```python
from build123d import *

# Parameters (mm, degrees)
SKETCH1_W               = 56
SKETCH1_H               = 4
BOSS_EXTRUDE1_DEPTH     = 168
SKETCH3_W               = 4
SKETCH3_H               = 32
BOSS_EXTRUDE4_DEPTH     = 4
LPATTERN2_COUNT         = 3
LPATTERN2_PITCH         = 50
MIRROR2_COPY_1_SKETCH_W = 4
MIRROR2_COPY_1_SKETCH_H = 32
MIRROR2_COPY_1_DEPTH    = 4
MIRROR2_COPY_2_SKETCH_W = 4
MIRROR2_COPY_2_SKETCH_H = 32
MIRROR2_COPY_2_DEPTH    = 4
SKETCH4_W               = 12
SKETCH4_H               = 4
BOSS_EXTRUDE5_DEPTH     = 4


with BuildPart() as part:
    # Sketch1 → Boss-Extrude1 (new body)
    with BuildSketch(Plane(origin=(0, 0, 0), x_dir=(1, 0, 0), z_dir=(0, 1, 0))):
        Rectangle(SKETCH1_W, SKETCH1_H)
    extrude(amount=BOSS_EXTRUDE1_DEPTH)

    # Sketch3 → Boss-Extrude4 (add, through all)
    with BuildSketch(Plane.XY.offset(2)):
        with Locations((-30, 34)):
            Rectangle(SKETCH3_W, SKETCH3_H)
    boss_extrude4 = extrude(amount=-BOSS_EXTRUDE4_DEPTH)

    # LPattern2: Boss-Extrude4 ×3
    with Locations(*[(0, i * LPATTERN2_PITCH, 0) for i in range(1, LPATTERN2_COUNT)]):
        add(boss_extrude4)

    # Mirror2: Boss-Extrude4 across plane
    add(boss_extrude4.mirror(Plane(origin=(0, 0, 0), x_dir=(0, 0, 1), z_dir=(1, 0, 0))))

    # Mirror2 copy 1 sketch → Mirror2 copy 1 (add, through all)
    with BuildSketch(Plane(origin=(0, 50, 2), x_dir=(-1, 0, 0), z_dir=(0, 0, 1))):
        with Locations((-30, -34)):
            Rectangle(MIRROR2_COPY_1_SKETCH_W, MIRROR2_COPY_1_SKETCH_H)
    extrude(amount=-MIRROR2_COPY_1_DEPTH)

    # Mirror2 copy 2 sketch → Mirror2 copy 2 (add, through all)
    with BuildSketch(Plane(origin=(0, 100, 2), x_dir=(-1, 0, 0), z_dir=(0, 0, 1))):
        with Locations((-30, -34)):
            Rectangle(MIRROR2_COPY_2_SKETCH_W, MIRROR2_COPY_2_SKETCH_H)
    extrude(amount=-MIRROR2_COPY_2_DEPTH)

    # Sketch4 → Boss-Extrude5 (add, through all)
    with BuildSketch(Plane.XY.offset(2)):
        with Locations((-22, 170)):
            Rectangle(SKETCH4_W, SKETCH4_H)
        with Locations((0, 170)):
            Rectangle(SKETCH4_W, SKETCH4_H)
        with Locations((22, 170)):
            Rectangle(SKETCH4_W, SKETCH4_H)
    boss_extrude5 = extrude(amount=-BOSS_EXTRUDE5_DEPTH)

    # Mirror3: Boss-Extrude5 across plane
    add(boss_extrude5.mirror(Plane.ZX.offset(84)))


solid = part.part
```
Can you work these out from the model? Positions are in its coordinate system, mm. A direction names the side the tool comes from. Give positions to 0.01 mm unless a question says otherwise; leave off trailing zeros. Loops run counter-clockwise (first coordinate to the right, second up) from the corner with the lowest first, then second, coordinate; pieces in that order, holes last. Notation, with made-up numbers: M -16,-9 L 15,-9 A26 cw 15,7 Z; hole C 37.5,89.25 d1. An arc over 180 degrees is marked long. Answer in a Markdown table with one row per item.
1. For pin 1 Ø2 at (y, z) = (-2, -0.5) entering from -X; pin 2 Ø2 at (x, z) = (31, 0.5) entering from +Y; pin 3 Ø1.2 at (x, z) = (30.5, 0) entering from -Y, each with a flat end and sliding along its axis, tell me the tip position at first contact or that it passes through.
Taken from the geometry:
| item | result |
|---|---|
| pin 1 | stops at x = -28 |
| pin 2 | stops at y = 150 |
| pin 3 | stops at y = 18 |
2. Suppose I cut it at A-A on x = -10. Write out the boundary of the cut face in (y, z), plus the area to 3 significant figures.
Taken from the geometry:
| item | result |
|---|---|
| outline | M 0,-2 L 168,-2 L 168,2 L 0,2 Z |
| area | 672 mm² |
3. Suppose I cut it at B-B on y = 113.5. Write out the boundary of the cut face in (x, z).
Taken from the geometry:
| item | result |
|---|---|
| outline | M -28,-2 L 28,-2 L 28,2 L -28,2 Z |
4. Which directions (+Z, -Z, +X, -X, +Y, -Y) give clear straight access to the entire face, cutting with the end or side of a thin tool? Please do faces 4 (the flat face through (-16, 170, 0)), 5 (the flat face through (-16, -2, 0)), 6 (the flat face through (30, 118, 0)), 7 (the flat face through (-28, 109, 0)).
Taken from the geometry:
| item | result |
|---|---|
| face 4 | +Z, -Z, +Y |
| face 5 | +Z, -Z, -Y |
| face 6 | +Z, -Z, +X |
| face 7 | +Z, -Z, -X |
5. If I drill on line 1 along Y through (x, z) = (28.5, 1.6); line 2 along X through (y, z) = (117, -0.55); line 3 along Y through (x, z) = (14, -0.8), over which ranges is the centre line in solid material (lowest first)?
Taken from the geometry:
| item | result |
|---|---|
| line 1 | y = 18 to 50, 68 to 100, 118 to 150 |
| line 2 | x = -28 to 28 |
| line 3 | y = 0 to 168 |
6. Thinking about a two-plate mould opening in X: for faces 1 (the flat face through (22, -4, 0)), 2 (the flat face through (11, 168, 0)), 3 (the flat face through (28, 109, 0)), which applies, released by +X, released by -X, zero draft, split by the parting line, or undercut?
Taken from the geometry:
| item | result |
|---|---|
| face 1 | zero draft |
| face 2 | undercut |
| face 3 | released by +X |
